Part print with two shaded views. Sizes in mm from the minimum x, y, z corner. A direction names the side the tool comes from. Give positions to 0.01 mm unless a question says otherwise; leave off trailing zeros. Order: outer loops, then holes, each group sorted by start corner. A loop starts at its lowest first (then second) coordinate and runs counter-clockwise, first axis right, second up. Notation, with made-up numbers: (54, 28.25) -> (112, 28.25) arc R20 ccw to (112, 48.25) -> close; hole circle Ø4 at (75.5, 79.25). An arc over 180 degrees is marked (long way). Answer as CSV lines item,"result".
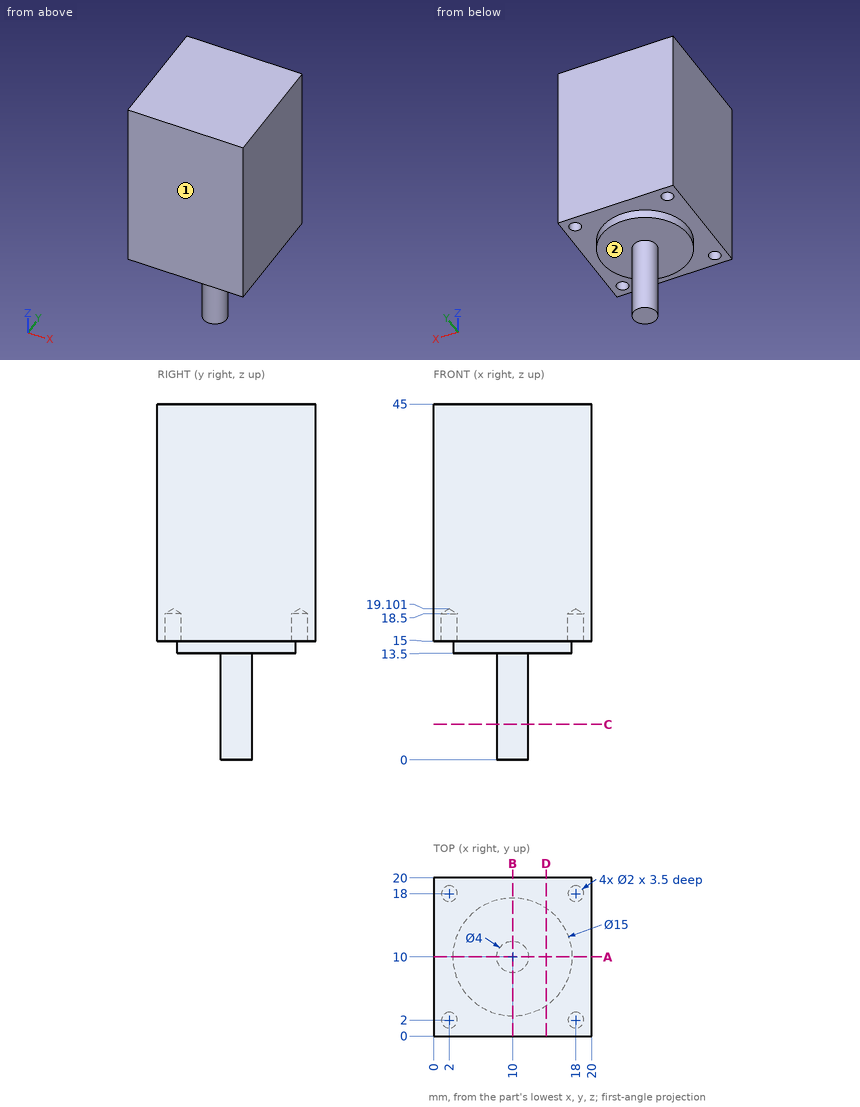
1) Pin check, flat tips, straight feed: P1, Ø5, axis at x = 15, y = 17.5, coming from the -Z side; P2, Ø3, axis at x = 2, y = 18, coming from the -Z side; P3, Ø1.2, axis at x = 2, y = 2, coming from the -Z side. Stop position of each tip, or through.
Data:
P1,"stops at z = 13.5"
P2,"stops at z = 15"
P3,"stops at z = 18.74"
2) Band-saw the part on A-A, the plane y = 10. Write the cut outline in (x, z), then the cut area to 4 significant figures.
Data:
outline,"(0, 15) -> (2.5, 15) -> (2.5, 13.5) -> (8, 13.5) -> (8, 0) -> (12, 0) -> (12, 13.5) -> (17.5, 13.5) -> (17.5, 15) -> (20, 15) -> (20, 45) -> (0, 45) -> close"
area,"676.5 mm2"
3) Which spindle directions (+Z, -Z, +X, -X, +Y, -Y) get a long thin tool onto all of the face, cutting with end or side? Do the marked faces 1 and 2. Say none if no direction does.
Data:
face 1,"+Z, -Z, +X, -X, -Y"
face 2,"-Z"
4) Wall check: line 1 along Y through (x, z) = (2, 16.55); line 2 along Z through (x, y) = (15, 6.75). Give the ranges that are in metal, low to high. Write a range as [from, to].
Data:
line 1,"y = [0, 1], [3, 17], [19, 20]"
line 2,"z = [13.5, 45]"
5) Band-saw the part on C-C, the plane z = 4.5. Write the cut outline in (x, y), then the cut area to 3 significant figures.
Data:
outline,"circle Ø4 at (10, 10)"
area,"12.6 mm2"
6) Band-saw the part on D-D, the plane x = 14.25. Write the cut outline in (y, z).
Data:
outline,"(0, 15) -> (3.82, 15) -> (3.82, 13.5) -> (16.18, 13.5) -> (16.18, 15) -> (20, 15) -> (20, 45) -> (0, 45) -> close"
